Autodesk Inventor part; units mm, degrees
ref_plane "YZ Plane" through (0, 0, 0) normal (1, 0, 0) x (0, 1, 0)
ref_plane "XZ Plane" through (0, 0, 0) normal (0, 1, 0) x (-1, 0, 0)
ref_plane "XY Plane" through (0, 0, 0) normal (0, 0, 1) x (1, 0, 0)
sketch "Szkic1" plane through (0, 0, 0) normal (0, 1, 0) x (-1, 0, 0)
  line L0 (0, 0) -> (44, 0)
  line L1 (44, 0) -> (44, -155)
  line L2 (44, -155) -> (0, -155)
  line L3 (0, -155) -> (0, 0)
  dimension "d0" = 44
  dimension "d1" = 155
extrude "Wyciągnięcie proste1" add sketch "Szkic1" along normal blind 25
sketch "Szkic2" plane through (-44, 0, 0) normal (0, 0, 1) x (1, 0, 0)
  line L0 (0, 0) -> (44, 0)
  line L1 (44, 0) -> (44, 25)
  line L2 (0, 25) -> (44, 25)
  line L3 (0, 0) -> (0, 25)
  line L4 (17.75, 20) -> (26.25, 20)
  line L5 (26.25, 20) -> (26.25, 5)
  line L6 (26.25, 5) -> (17.75, 5)
  line L7 (17.75, 5) -> (17.75, 20)
  circle A0 centre (22, 17.25) radius 2.75
  circle A1 centre (22, 7.75) radius 2.75
  point P0 (26.25, 12.5)
  point P1 (44, 12.5)
  point P2 (22, 20)
  point P3 (22, 25)
  point P4 (22, 5)
  point P5 (22, 20)
  point P6 (22, 5)
  dimension "d4" = 8.5
  dimension "d5" = 15
  dimension "d6" = 5.5
  dimension "d7" = 5.5
extrude "Wyciągnięcie proste2" cut sketch "Szkic2" against normal blind 1 contours L4 L5 L6 L7
extrude "Wyciągnięcie proste3" add sketch "Szkic2" along normal blind 5 contours A1 | A0
properties part number "li_pol_3S_5000mAh"
Geometry check sheet. Reference: the model listing, model coordinates, mm. Give positions to 0.01 mm unless a question says otherwise; leave off trailing zeros. Order: outer loops, then holes, each group sorted by start corner. A loop starts at its lowest first (then second) coordinate and runs counter-clockwise, first axis right, second up. Notation, with made-up numbers: (48.25, 49.5) - (77.25, 49.5) arc R21 cw to (77.25, 80.5) - close; hole circle Ø10 at (45.25, 7.5). An arc over 180 degrees is marked (long way). Write item = value, one per line. Start each with the question number.
1) Draft check along Y on faces 1 (the flat face through (-22, 17, 5)), 2 (the flat face through (-22, 25, -76)), 3 (the flat face through (-22, 13, -1)). Enter one of: released by +Y, released by -Y, zero draft, split by the parting line, or undercut.
2) Section check B-B (x = -30). Enter the section's corners in (y, z), then the cut area to 4 significant figures.
3) Section check A-A (y = 12.75). Enter the section's corners in (x, z).
4) Scan lines: L1, parallel to Z at x = -5.5, y = 3; L2, parallel to Z at x = -25, y = 13.25. Record each from-to range of solid material in increasing order.
Geometry check:
q1.face_1 = zero draft
q1.face_2 = released by +Y
q1.face_3 = undercut
q2.outline = (0, -155) - (25, -155) - (25, 0) - (0, 0) - close
q2.area = 3,875 mm2
q3.outline = (-44, -155) - (0, -155) - (0, 0) - (-17.75, 0) - (-17.75, -1) - (-26.25, -1) - (-26.25, 0) - (-44, 0) - close
q4.L1 = -155 to 0
q4.L2 = -155 to -1
